The listing builds one solid part. Answer for the finished solid, in the listing's coordinates (mm). A direction names the side the tool comes from. Give positions to 0.01 mm unless a question says otherwise; leave off trailing zeros. Write each loop counter-clockwise with the first axis right and the second up, starting at its lowest first coordinate (ties: lowest second). Pieces come first, ordered by that corner, then holes. Notation, with made-up numbers: (41.5, -16) -> (70.5, -16) arc R21 ccw to (70.5, 5) -> close; hole circle Ø9 at (67.25, -29.5). An arc over 180 degrees is marked (long way). Write each question's results on one line, items separated by ' | '. Start each with the question number.
from build123d import *

# Parameters (mm, degrees)
SKETCH_1_W               = 22
SKETCH_1_H               = 20
EXTRUDE_1_DEPTH          = 13
SKETCH_2_W               = 15.9
SKETCH_2_H               = 22.004551976
EXTRUDE_2_DEPTH          = 3
SKETCH_3_W               = 22
SKETCH_3_H               = 5.5
EXTRUDE_3_DEPTH          = 4.1
EXTRUDE_4_DEPTH          = 8
EXTRUDE_5_DEPTH          = 8
SKETCH_7_R               = 1.5
CUT_EXTRUDE_1_DEPTH      = 5
CUT_EXTRUDE_2_DEPTH      = 35.799425283
CUT_EXTRUDE_2_DEPTH_BACK = 9
SKETCH_9_R               = 3.95


with BuildPart() as part:
    # 草图1 → 凸台-拉伸1 (new body)
    with BuildSketch(Plane(origin=(0, 0, 0), x_dir=(0, 0, -1), z_dir=(1, 0, 0))):
        Rectangle(SKETCH_1_W, SKETCH_1_H)
    extrude(amount=EXTRUDE_1_DEPTH)

    # 草图2 → 凸台-拉伸2 (add)
    with BuildSketch(Plane(origin=(0, 10, 0), x_dir=(1, 0, 0), z_dir=(0, 1, 0))):
        with Locations((7.95, 0.002275988)):
            Rectangle(SKETCH_2_W, SKETCH_2_H)
    extrude(amount=EXTRUDE_2_DEPTH)

    # 草图3 → 凸台-拉伸3 (add)
    with BuildSketch(Plane(origin=(15.9, 0, 0), x_dir=(0, 0, -1), z_dir=(1, 0, 0))):
        with Locations((0, 10.25)):
            Rectangle(SKETCH_3_W, SKETCH_3_H)
    extrude(amount=EXTRUDE_3_DEPTH)

    # 草图5 → 凸台-拉伸4 (add)
    with BuildSketch(Plane.XY.offset(11)):
        Polygon((13, 13), (13, 10), (15.9, 10), (15.9, 7.5), (20, 7.5), (20, 13), align=None)
    extrude(amount=EXTRUDE_4_DEPTH)

    # 草图6 → 凸台-拉伸5 (add)
    with BuildSketch(Plane(origin=(0, 0, -11), x_dir=(-1, 0, 0), z_dir=(0, 0, -1))):
        Polygon((-13, 13), (-13, 10), (-15.9, 10), (-15.9, 7.5), (-20, 7.5), (-20, 13), align=None)
    extrude(amount=EXTRUDE_5_DEPTH)

    # 草图7 → 切除-拉伸1 (cut)
    with BuildSketch(Plane(origin=(13, 0, 0), x_dir=(0, 0, -1), z_dir=(1, 0, 0))):
        with Locations((0, 2.1)):
            Circle(SKETCH_7_R)
    extrude(amount=-CUT_EXTRUDE_1_DEPTH, mode=Mode.SUBTRACT)

    # 草图9 → 切除-拉伸2 (cut, two sides: drawn at the far end of the back side and taken through both)
    with BuildSketch(Plane(origin=(-5, 5, 0), x_dir=(0, 0, -1), z_dir=(-0.7071067811865464, 0.7071067811865488, 0)).offset(-CUT_EXTRUDE_2_DEPTH_BACK)):
        with Locations(Location((0, -11.341614651, 0), (0, 0, 147.03627328))):
            Circle(SKETCH_9_R)
    extrude(amount=CUT_EXTRUDE_2_DEPTH + CUT_EXTRUDE_2_DEPTH_BACK, mode=Mode.SUBTRACT)


solid = part.part
1. Each of these flat-tipped pins is pushed along its axis until it touches: pin 1 Ø6.5 at (x, y) = (3.5, 5) entering from -Z; pin 2 Ø1.2 at (x, z) = (18.5, 3.5) entering from -Y; pin 3 Ø0.9 at (y, z) = (11, -13.5) entering from -X. Where does it stop, or does it pass through?
2. Section D-D (z = -13.5) is taken. Write down the section's boundary in (x, y), then the cut area to 4 significant figures.
3. A tool of negligible diameter and unlimited length cuts with its end or side. For faces 1 (the flat face through (6, 11, -11.005)), 2 (the flat face through (15.9, 9, 0)), 3 (the cylindrical face through (10.535, 3.587, 0.195)), 4 (the flat face through (13, 12, 15)), from which of +Z, -Z, +X, -X, +Y, -Y can it reach the whole face along a straight path? Write none if from no direction.
4. Section C-C (x = 18) is taken. Write down the section's boundary in (y, z), then the cut area to 3 significant figures.
5. The mould has two halves that part along Y. Classify faces 5 (the flat face through (13, 12, -15)), 6 (the flat face through (18, 7.5, 0)), 7 (the flat face through (8, 2, 0)): pulls with the +Y half, pulls with the -Y half, needs draft (parallel to the pull), parting line crosses it, or undercut.
6. Section B-B (y = 2.1) is taken. Write down the section's boundary in (x, z).
7. Section A-A (z = -5) is taken. Write down the section's boundary in (x, y).
8. Consider probe 1 along Y at (x, z) = (11.7, 0); probe 2 along X at (y, z) = (-6.25, 1); probe 3 along X at (y, z) = (10.5, -13.5). Determine where each line is inside the solid, lowest interval first. Write a range as [from, to].
Results:
1) pin 1: stops at z = -11 | pin 2: stops at y = 7.5 | pin 3: stops at x = 13
2) outline: (13, 10) -> (15.9, 10) -> (15.9, 7.5) -> (20, 7.5) -> (20, 13) -> (13, 13) -> close | area: 31.25 mm²
3) face 1: -Z, -X, +Y, -Y | face 2: +Z, -Z, -Y | face 3: +X | face 4: +Z, -X, +Y, -Y
4) outline: (7.5, -19) -> (13, -19) -> (13, 19) -> (7.5, 19) -> close | area: 209 mm²
5) face 5: needs draft | face 6: pulls with the -Y half | face 7: undercut
6) outline: (0, -11) -> (13, -11) -> (13, -1.5) -> (8, -1.5) -> (8, 1.5) -> (13, 1.5) -> (13, 11) -> (0, 11) -> close
7) outline: (0, -10) -> (13, -10) -> (13, 10) -> (15.9, 10) -> (15.9, 7.5) -> (20, 7.5) -> (20, 13) -> (0, 13) -> close
8) probe 1: y = [-10, 0.6], [3.6, 8.97], [9.93, 13] | probe 2: x = [0, 13] | probe 3: x = [13, 20]
